Read the model definition and answer for the solid it produces. Units are mm, in the model's axes. A direction names the side the tool comes from. Round coordinates to 2 decimals unless told otherwise and drop trailing zeros. Loops run counter-clockwise (first coordinate to the right, second up) from the corner with the lowest first, then second, coordinate; pieces in that order, holes last. Notation, with made-up numbers: M 11,35.25 L 63,35.25 A14 cw 63,56.25 Z; hole C -19,23 d2. An arc over 180 degrees is marked long. Write each question's results on one line, items separated by ' | '.
```python
from build123d import *

# Parameters (mm, degrees)
F4_DEPTH = 300


with BuildPart() as f4:
    # F3 (on offset) → F4 (new body)
    with BuildSketch(Plane.XZ.offset(25)):
        Polygon((-168.0019225023, 96.9915152759), (-150.0017165199, 86.5995672107), (0, 173.2070629141), (0, 193.9919104638), align=None)
    extrude(amount=F4_DEPTH)

    # F5: F4 across face


with BuildPart() as f4_1:
    add(f4.part)
    add(f4.part.mirror(Plane(origin=(0, -175, 183.599486689), x_dir=(0, 1, 0), z_dir=(1, 0, 0))))

    # F6: F4 across face


with BuildPart() as f4_2:
    add(f4_1.part)
    add(f4_1.part.mirror(Plane(origin=(159.0018195111, -175, 91.7955412433), x_dir=(0, 1, 0), z_dir=(0.4999828344, 0, -0.8660353141))))

    # F7: F4 across face


with BuildPart() as f4_3:
    add(f4_2.part)
    add(f4_2.part.mirror(Plane(origin=(-159.0018195111, -175, 91.7955412433), x_dir=(0, -1, 0), z_dir=(-0.4999828344, 0, -0.8660353141))))


solid = f4_3.part
```
1. Find section A-A, the plane z = -45.5. Give the vertices of the cut face in (x, y), then the cut area to 3 significant figures.
Completed:
outline: M -168,-325 L -150,-325 L -150,-25 L -168,-25 Z; M 150,-325 L 168,-325 L 168,-25 L 150,-25 Z | area: 10,800 mm2
2. Given P1, Ø8, axis at y = -248.5, z = 147, coming from the +X side; P2, Ø8, axis at y = -102.5, z = -141, coming from the -X side; P3, Ø10, axis at y = -255.5, z = -68, coming from the -X side, each flat-ended and moving along its own axis, determine where each tip first touches the part or whether it passes through.
Completed:
P1: stops at x = 88.32 | P2: stops at x = -98.71 | P3: stops at x = -168
3. Determine the mould class of faces 1 (the face through (-82.825, -172.9, 146.171)), 2 (the face through (-76.051, -172.9, 129.297)), 3 (the face through (-85.2, -172.9, -144.8)) for opening direction Z: released by +Z, released by -Z, zero draft, split by the parting line, or undercut.
Completed:
face 1: released by +Z | face 2: undercut | face 3: released by -Z
4. Find the intervals of material crossed by L1, parallel to X at y = -267.5, z = -26; L2, parallel to Z at x = -126.5, y = -279.5; L3, parallel to Z at x = 32, y = -249.5, in increasing order.
Completed:
L1: x = -168 to -150, 150 to 168 | L2: z = -120.96 to -100.17, 100.17 to 120.95 | L3: z = -175.52 to -154.73, 154.73 to 175.52
5. Which of the six approach directions +Z, -Z, +X, -X, +Y, -Y give full straight-line access (tool end or side, diameter ignored) to faces 4 (the face through (-74.3, -25, -130.5)), 5 (the face through (76.046, -172.9, 129.3))?
Completed:
face 4: +Z, -Z, +X, -X, +Y | face 5: +Y, -Y
6. Find section C-C, the plane x = 108. Give the vertices of the cut face in (y, z).
Completed:
outline: M -325,-131.64 L -25,-131.64 L -25,-110.85 L -325,-110.85 Z; M -325,110.85 L -25,110.85 L -25,131.64 L -325,131.64 Z
